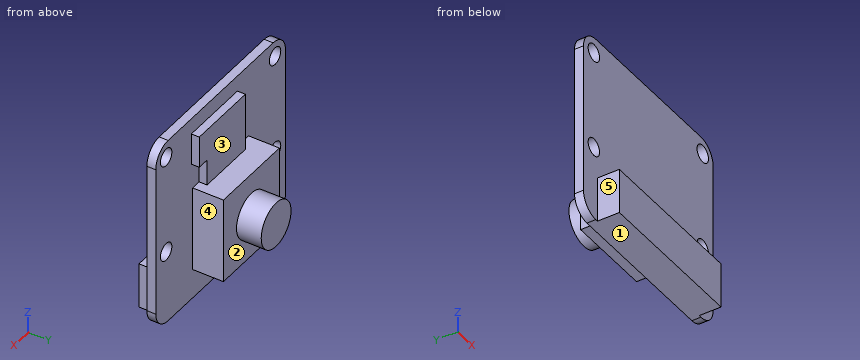
from build123d import *

# Parameters (mm, degrees)
MAINBOARD_DEPTH     = 1.12
SKETCH2_R           = 1.1
BOARDHOLES_DEPTH    = 1.12
CAMBOD_W            = 10.8
CAMBOD_H            = 10.8
CAM_BASE_DEPTH      = 3.875
CAMLENS_START       = -3.875
SKETCH4_R           = 2.875
CAMLENS_DEPTH       = 6.98
SKETCH5_W           = 19.61
SKETCH5_H           = 5.71
RIBBON_PORT_DEPTH   = 2.75
LITTLE_MODULE_DEPTH = 1


with BuildPart() as part:
    # Sketch1 → MainBoard (new body)
    with BuildSketch(Plane(origin=(0, 0, 0), x_dir=(1, 0, 0), z_dir=(0, 1, 0))):
        with BuildLine():
            Line((-10.125, 11.931), (10.125, 11.931))
            ThreePointArc((10.125, 11.931), (11.804378605, 11.235378605), (12.5, 9.556))
            Line((12.5, 9.556), (12.5, -9.556))
            ThreePointArc((12.5, -9.556), (11.804378605, -11.235378605), (10.125, -11.931))
            Line((10.125, -11.931), (-10.125, -11.931))
            ThreePointArc((-10.125, -11.931), (-11.804378605, -11.235378605), (-12.5, -9.556))
            Line((-12.5, -9.556), (-12.5, 9.556))
            ThreePointArc((-12.5, 9.556), (-11.804378605, 11.235378605), (-10.125, 11.931))
        make_face()
    extrude(amount=MAINBOARD_DEPTH)

    # Sketch2 → BoardHoles (cut)
    with BuildSketch(Plane(origin=(0, 1.12, 0), x_dir=(1, 0, 0), z_dir=(0, 1, 0))):
        with Locations(Location((-10.5, -9.931, 0), (0, 0, 270))):
            Circle(SKETCH2_R)
        with Locations(Location((-10.5, 2.569, 0), (0, 0, 270))):
            Circle(SKETCH2_R)
        with Locations(Location((10.5, -9.931, 0), (0, 0, 270))):
            Circle(SKETCH2_R)
        with Locations(Location((10.5, 2.569, 0), (0, 0, 270))):
            Circle(SKETCH2_R)
    extrude(amount=-BOARDHOLES_DEPTH, mode=Mode.SUBTRACT)

    # CamBod → Cam Base (add)
    with BuildSketch(Plane(origin=(0, 1.12, 0), x_dir=(1, 0, 0), z_dir=(0, 1, 0))):
        with Locations((0, 2.769)):
            Rectangle(CAMBOD_W, CAMBOD_H)
    extrude(amount=CAM_BASE_DEPTH)

    # Sketch4 → CamLens (add)
    with BuildSketch(Plane(origin=(0, 4.995, 0), x_dir=(1, 0, 0), z_dir=(0, 1, 0)).offset(CAMLENS_START)):
        with Locations(Location((0, 2.769, 0), (0, 0, 270))):
            Circle(SKETCH4_R)
    extrude(amount=CAMLENS_DEPTH)

    # Sketch5 → Ribbon Port (add)
    with BuildSketch(Plane.XZ):
        with Locations((0, -9.076)):
            Rectangle(SKETCH5_W, SKETCH5_H)
    extrude(amount=RIBBON_PORT_DEPTH)

    # Sketch6 → Little Module (add)
    with BuildSketch(Plane(origin=(0, 1.12, 0), x_dir=(1, 0, 0), z_dir=(0, 1, 0))):
        Polygon((-3.25, -9.931), (-3.25, -2.631), (4.15, -2.631), (4.15, -5.931), (5.65, -5.931), (5.65, -9.931), align=None)
    extrude(amount=LITTLE_MODULE_DEPTH)


solid = part.part
Read the model definition and answer for the solid it produces. Units are mm, in the model's axes. Face numbers are marked on the shaded views. A direction names the side the tool comes from. Round coordinates to 2 decimals unless told otherwise and drop trailing zeros. Loops run counter-clockwise (first coordinate to the right, second up) from the corner with the lowest first, then second, coordinate; pieces in that order, holes last.
Q1. Consider probe 1 along X at (y, z) = (-2, -8) (3 decimals); probe 2 along Y at (x, z) = (5.5, 7.5); probe 3 along Z at (x, y) = (-1, -0.5). Determine where each line is inside the solid, lowest interval first.
Q2. Section B-B on x = 7.5 is taken. Write down the section's boundary in (y, z).
Q3. Each of these flat-tipped pins is pushed along its axis until it touches: pin 1 (3.5 mm diameter, centred on x = -10.5, z = -2.569, fed in from -Y); pin 2 (1 mm diameter, centred on x = -7.5, y = -1, fed in from +Z); pin 3 (1.9 mm diameter, centred on x = 0.5, y = 2.5, fed in from +Z). Where does it stop, or does it pass through?
Q4. Section D-D on y = -1.75 is taken. Write down the section's boundary in (x, z) (3 decimals).
Q5. Section A-A on z = -2 is taken. Write down the section's boundary in (x, y) (3 decimals), and give its area (3 significant figures).
Q6. Section C-C on x = -10.5 is taken. Write down the section's boundary in (y, z).
Q7. Which of the six approach directions +Z, -Z, +X, -X, +Y, -Y give full straight-line access (tool end or side, diameter ignored) to the marked faces 1, 2, 3, 4 and 5?
Output:
1. probe 1: x = -9.805 to 9.805
1. probe 2: y = 0 to 2.12
1. probe 3: z = -11.93 to -6.22
2. outline: (-2.75, -11.93) - (1.12, -11.93) - (1.12, 11.93) - (0, 11.93) - (0, -6.22) - (-2.75, -6.22) - close
3. pin 1: stops at y = 0
3. pin 2: stops at z = -6.22
3. pin 3: stops at z = 9.93
4. outline: (-9.805, -11.931) - (9.805, -11.931) - (9.805, -6.221) - (-9.805, -6.221) - close
5. outline: (-12.5, 0) - (-11.441, 0) - (-11.441, 1.12) - (-12.5, 1.12) - close; (-9.559, 0) - (9.559, 0) - (9.559, 1.12) - (5.4, 1.12) - (5.4, 4.995) - (2.77, 4.995) - (2.77, 8.1) - (-2.77, 8.1) - (-2.77, 4.995) - (-5.4, 4.995) - (-5.4, 1.12) - (-9.559, 1.12) - close; (11.441, 0) - (12.5, 0) - (12.5, 1.12) - (11.441, 1.12) - close
5. area: 82.8 mm2
6. outline: (0, -11.9) - (1.12, -11.9) - (1.12, -3.67) - (0, -3.67) - close; (0, -1.47) - (1.12, -1.47) - (1.12, 8.83) - (0, 8.83) - close; (0, 11.03) - (1.12, 11.03) - (1.12, 11.9) - (0, 11.9) - close
7. face 1: -Z, +X, -X, +Y, -Y
7. face 2: +Y
7. face 3: +Z, +X, -X, +Y
7. face 4: -Z, +X, +Y
7. face 5: +Z, -Z, -X, -Y
